Check sheet for the modelled part. Datum: model origin and axes. Units: mm. Face numbers are marked on the shaded views. A direction names the side the tool comes from. Round coordinates to 2 decimals unless told otherwise and drop trailing zeros. Write each loop counter-clockwise with the first axis right and the second up, starting at its lowest first coordinate (ties: lowest second). Pieces come first, ordered by that corner, then holes.
Item 1: Release check for a two-part mould opening along Y. For the marked faces 1, 2 and 3 record: pulls with the +Y half, pulls with the -Y half, needs draft (parallel to the pull), parting line crosses it, or undercut.
Item 2: Material ranges on line 1 along Z through (x, y) = (-51, -1.75); line 2 along Y through (x, z) = (-63, 17); line 3 along Z through (x, y) = (-39, 1.75), recorded low to high.
Item 3: Section check B-B, the plane z = -11.15. Record the cut outline in (x, y).
Item 4: Section check A-A, the plane z = 3. Record the cut outline in (x, y).
Item 5: Section check C-C, the plane x = -29. State how many separate pieces and enclosed holes the cut face has, plus the area to 3 significant figures.
Item 6: Section check D-D, the plane z = -2.5. Record the cut outline in (x, y).
Item 7: Depth check by flat-ended pin: pin 1 (1.2 mm diameter, centred on x = -5.5, y = 22, fed in from -Z); pin 2 (13 mm diameter, centred on x = -43.5, z = 31.5, fed in from +Y); pin 3 (4.5 mm diameter, centred on x = -8, y = 22.5, fed in from +Z); pin 4 (6 mm diameter, centred on y = 14.5, z = 29, fed in from -X). Enter the tip coordinate at first touch or a pass-through.
Item 8: Set-up check for the marked faces 4 and 5: record each of +Z, -Z, +X, -X, +Y, -Y from which the full face is reachable in a straight line by a thin tool's end or side.
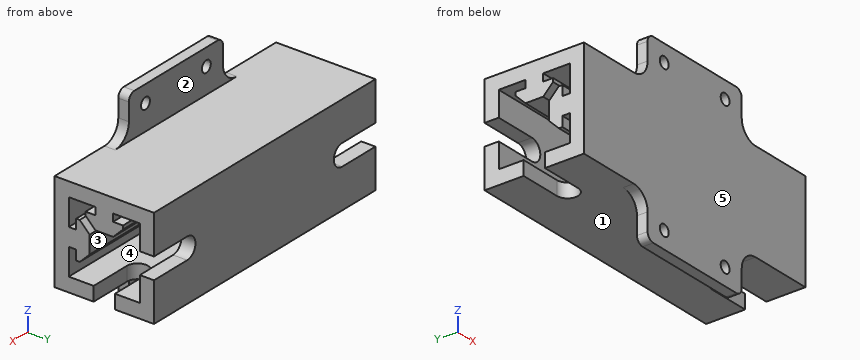
Autodesk Inventor part; units mm, degrees
ref_plane "YZ Plane" through (0, 0, 0) normal (1, 0, 0) x (0, 1, 0)
ref_plane "XZ Plane" through (0, 0, 0) normal (0, 1, 0) x (-1, 0, 0)
ref_plane "XY Plane" through (0, 0, 0) normal (0, 0, 1) x (1, 0, 0)
sketch "Sketch1" plane through (0, 0, 0) normal (1, 0, 0) x (0, 1, 0)
  line L0 (0, 0) -> (20.1, 0)
  line L1 (20.1, 0) -> (20.1, 20.1)
  line L2 (20.1, 20.1) -> (0, 20.1)
  line L3 (0, 20.1) -> (0, 0)
  line L4 (-4, 24.1) -> (24.1, 24.1)
  line L5 (24.1, 24.1) -> (24.1, -4)
  line L6 (24.1, -4) -> (-4, -4)
  line L7 (-4, -4) -> (-4, 24.1)
  line L8 (12.55, 22.2) -> (7.55, 22.2)
  line L9 (7.55, 22.2) -> (7.55, 18)
  line L10 (7.55, 18) -> (12.55, 18)
  line L11 (12.55, 18) -> (12.55, 22.2)
  line L12 (12.55, 22.2) -> (7.55, 18) construction
  line L13 (7.55, 22.2) -> (12.55, 18) construction
  line L14 (12.55, 18) -> (15.35, 18)
  line L15 (15.35, 18) -> (15.35, 17)
  line L16 (15.35, 17) -> (12.55, 14.2)
  line L17 (12.55, 14.2) -> (7.55, 14.2)
  line L18 (7.55, 18) -> (4.75, 18)
  line L19 (4.75, 18) -> (4.75, 17)
  line L20 (4.75, 17) -> (7.55, 14.2)
  line L21 (2.1, 15.35) -> (3.1, 15.35)
  line L22 (3.1, 4.75) -> (5.9, 7.55)
  line L23 (2.1, 4.75) -> (3.1, 4.75)
  line L24 (-2.1, 12.55) -> (-2.1, 7.55)
  line L25 (2.1, 12.55) -> (-2.1, 12.55)
  line L26 (-2.1, 12.55) -> (2.1, 7.55) construction
  line L27 (-2.1, 7.55) -> (2.1, 12.55) construction
  line L28 (2.1, 7.55) -> (2.1, 4.75)
  line L29 (-2.1, 7.55) -> (2.1, 7.55)
  line L30 (2.1, 7.55) -> (2.1, 12.55)
  line L31 (5.9, 12.55) -> (5.9, 7.55)
  line L32 (2.1, 12.55) -> (2.1, 15.35)
  line L33 (3.1, 15.35) -> (5.9, 12.55)
  point P0 (10.05, 20.1)
  point P1 (0, 10.05)
  point P2 (10.05, 20.1)
  point P3 (0, 10.05)
  point P4 (0, 7.55)
  point P5 (0, 12.55)
  point P6 (7.55, 20.1)
  point P7 (12.55, 20.1)
  dimension "d0" = 20.1
  dimension "d1" = 20.1
  dimension "d2" = 4
  dimension "d3" = 5
  dimension "d4" = 4.2
  dimension "d5" = 2.8
  dimension "d6" = 1
  dimension "d7" = 3.8
  dimension "d8" = 2.8
  dimension "d9" = 5
  dimension "d10" = 1
  dimension "d11" = 135
  dimension "d12" = 5
  dimension "d13" = 4.2
  dimension "d14" = 2.8
  dimension "d15" = 1
  dimension "d16" = 3.8
  dimension "d17" = 2.8
  dimension "d18" = 5
  dimension "d19" = 1
  dimension "d20" = 135
  dimension "d21" = 7.55
  dimension "d22" = 2.1
  dimension "d23" = 90
  dimension "d24" = 7.55
  dimension "d25" = 2.1
  dimension "d26" = 90
extrude "Extrusion1" add sketch "Sketch1" against normal blind 80 contours L29 L24 L25 L3 | L3 L25 L30 L29 | L30 L32 L21 L33 L31 L22 L23 L28 | L11 L10 L9 L2 | L2 L9 L8 L11 | L14 L15 L16 L17 L20 L19 L18 L10 | L4 L5 L6 L7
sketch "Sketch2" plane through (0, -4, -4) normal (0, -1, 0) x (1, 0, 0)
  line L0 (0, 28.1) -> (0, 0)
  line L1 (0, 28.1) -> (-80, 28.1)
  line L2 (-80, 0) -> (-80, 28.1)
  line L3 (0, 0) -> (-80, 0)
  line L4 (-80, 0) -> (0, 28.1) construction
  line L5 (-80, 28.1) -> (0, 0) construction
  line L6 (-51, 35.25) -> (-51, -7.15) construction
  line L7 (-51, -7.15) -> (-29, -7.15) construction
  line L8 (-29, -7.15) -> (-29, 35.25) construction
  line L9 (-29, 35.25) -> (-51, 35.25) construction
  line L10 (-51, 35.25) -> (-29, -7.15) construction
  line L11 (-51, -7.15) -> (-29, 35.25) construction
  circle A0 centre (-29, 35.25) radius 1.6
  circle A1 centre (-29, -7.15) radius 1.6
  circle A2 centre (-51, 35.25) radius 1.6
  circle A3 centre (-51, -7.15) radius 1.6
  line L12 (-23, 28.1) -> (-57, 28.1)
  line L13 (-57, 28.1) -> (-57, 40.1)
  line L14 (-57, 40.1) -> (-23, 40.1)
  line L15 (-23, 40.1) -> (-23, 28.1)
  line L16 (-23, 0) -> (-57, 0)
  line L17 (-57, 0) -> (-57, -12)
  line L18 (-57, -12) -> (-23, -12)
  line L19 (-23, -12) -> (-23, 0)
  point P0 (0, 4)
  point P1 (-40, 14.05)
  dimension "d29" = 42.4
  dimension "d31" = 22
  dimension "d32" = 3.2
  dimension "d35" = 42.4
  dimension "d38" = 22
  dimension "d41" = 34
  dimension "d42" = 12
  dimension "d43" = 6
  dimension "d44" = 12
  dimension "d45" = 6
  dimension "d46" = 34
extrude "Extrusion2" add sketch "Sketch2" against normal blind 3 contours L1 L13 L14 L15 | L19 L18 L17 L3
sketch "Sketch3" plane through (0, 24.1, 24.1) normal (0, 1, 0) x (1, 0, 0)
  line L0 (0, 28.1) -> (0, 0)
  line L1 (0, 28.1) -> (-80, 28.1)
  line L2 (-80, 0) -> (-80, 28.1)
  line L3 (0, 0) -> (-80, 0)
  line L4 (0, 16.55) -> (0, 11.55) construction
  line L5 (0, 14.05) -> (-80, 14.05) construction
  line L6 (-80, 28.1) -> (-80, 0) construction
  circle A0 centre (-12, 14.05) radius 3
  circle A1 centre (-68, 14.05) radius 3
  line L7 (-68, 17.05) -> (-80, 17.05)
  line L8 (-68, 11.05) -> (-80, 11.05)
  line L9 (-12, 17.05) -> (0, 17.05)
  line L10 (0, 19.35) -> (0, 16.55)
  line L11 (-12, 11.05) -> (0, 11.05)
  line L12 (0, 8.75) -> (0, 11.55)
  point P0 (0, 24.1)
  point P1 (0, 11.05)
  point P2 (-80, 11.05)
  dimension "d49" = 6
  dimension "d50" = 6
  dimension "d51" = 12
  dimension "d52" = 12
  dimension "d53" = 6
  dimension "d54" = 6
extrude "Extrusion3" cut sketch "Sketch3" against normal up to surface (4 mm away) contours L0 L11 A0 L9 | L7 A1 L8 L2 | A0 | A1
ref_plane "Work Plane1" through (0, 24.1, -4) normal (0, -0.7071, -0.7071) x (-1, 0, 0)
mirror "Mirror1" about plane through (0, 24.1, -4) normal (0, -0.7071, -0.7071) of "Extrusion3"
fillet "Fillet1" radius 2 4 edges at (-23, -2.5, -16) (-57, -2.5, -16) (-57, -2.5, 36.1) (-23, -2.5, 36.1)
fillet "Fillet2" radius 5 4 edges at (-23, -2.5, -4) (-57, -2.5, -4) (-57, -2.5, 24.1) (-23, -2.5, 24.1)
equation "\"d8\" = d5"
equation "\"d9\" = d3"
equation "\"d10\" = d6"
equation "\"d17\" = d14"
equation "\"d18\" = d12"
equation "\"d19\" = d15"
properties part number "cameraSlider"
Values found:
1. face 1: needs draft
1. face 2: pulls with the +Y half
1. face 3: undercut
2. line 1: z = -16 to -12.75, -9.55 to 29.65, 32.85 to 36.1
2. line 2: y = -4 to 0, 4.75 to 15.35, 20.1 to 24.1
2. line 3: z = -4 to 0, 7.55 to 12.55, 20.1 to 24.1
3. outline: (-57, -4) - (-52.6, -4) - (-52.6, -1) - (-57, -1) - close; (-49.4, -4) - (-30.6, -4) - (-30.6, -1) - (-49.4, -1) - close; (-27.4, -4) - (-23, -4) - (-23, -1) - (-27.4, -1) - close
4. outline: (-80, -4) - (0, -4) - (0, 0) - (-80, 0) - close; (-80, 20.1) - (0, 20.1) - (0, 24.1) - (-80, 24.1) - close
5. separate pieces: 3
5. enclosed holes: 1
5. area: 524 mm2
6. outline: (-80, -4) - (0, -4) - (0, 7.05) - (-12, 7.05) arc R3 cw to (-12, 13.05) - (0, 13.05) - (0, 24.1) - (-80, 24.1) - (-80, 13.05) - (-68, 13.05) arc R3 cw to (-68, 7.05) - (-80, 7.05) - close
7. pin 1: stops at z = -4
7. pin 2: stops at y = -1
7. pin 3: stops at z = 24.1
7. pin 4: passes through
8. face 4: +X, -X
8. face 5: +Z, -Z, +X, -X, -Y
